from build123d import *

# Parameters (mm, degrees)
CROQUIS1_W              = 304.8
CROQUIS1_H              = 228.6
SALIENTE_EXTRUIR1_DEPTH = 1500
VACIADO1_T              = -2
CROQUIS2_W              = 25.4
CROQUIS2_H              = 228.6
CROQUIS2_W_2            = 304.8
CROQUIS2_H_2            = 25.4
SALIENTE_EXTRUIR2_DEPTH = 2


with BuildPart() as part:
    # Croquis1 → Saliente-Extruir1 (new body)
    with BuildSketch(Plane(origin=(0, 0, 0), x_dir=(1, 0, 0), z_dir=(0, 1, 0))):
        Rectangle(CROQUIS1_W, CROQUIS1_H)
    extrude(amount=SALIENTE_EXTRUIR1_DEPTH)

    # Vaciado1
    vaciado1_openings = [part.faces().sort_by_distance(p)[0] for p in [
        (0, 1500, 0),
        (0, 0, 0),
    ]]
    offset(amount=VACIADO1_T, openings=vaciado1_openings, kind=Kind.INTERSECTION)

    # Croquis2 → Saliente-Extruir2 (add)
    with BuildSketch(Plane(origin=(0, 1500, 0), x_dir=(1, 0, 0), z_dir=(0, 1, 0))):
        with Locations((-165.1, 0)):
            Rectangle(CROQUIS2_W, CROQUIS2_H)
        with Locations((0, 127)):
            Rectangle(CROQUIS2_W_2, CROQUIS2_H_2)
        with Locations((0, -127)):
            Rectangle(CROQUIS2_W_2, CROQUIS2_H_2)
        with Locations((165.1, 0)):
            Rectangle(CROQUIS2_W, CROQUIS2_H)
    saliente_extruir2 = extrude(amount=-SALIENTE_EXTRUIR2_DEPTH)

    # Simetría1: Saliente-Extruir2 across plane
    add(saliente_extruir2.mirror(Plane.ZX.offset(750)))


solid = part.part
CAD build for the part. Positions are in the model's coordinates, mm. A direction names the side the tool comes from. Give positions to 0.01 mm unless a question says otherwise; leave off trailing zeros. Loops run counter-clockwise (first coordinate to the right, second up) from the corner with the lowest first, then second, coordinate; pieces in that order, holes last. Notation, with made-up numbers: M 34.5,-28.5 L 43.5,-28.5 A27 cw 43.5,8.5 Z; hole C -22,5.25 d5. An arc over 180 degrees is marked long. Write each question's results on one line, items separated by ' | '.
Q1. Band-saw the part on C-C on y = 432. Write the cut outline in (x, z).
Geometry check:
outline: M -152.4,-114.3 L 152.4,-114.3 L 152.4,114.3 L -152.4,114.3 Z; hole M -150.4,-112.3 L 150.4,-112.3 L 150.4,112.3 L -150.4,112.3 Z
Q2. Probe probe 1 along Z at (x, y) = (-106.5, 1095.5); probe 2 along X at (y, z) = (127, 27). List the from-to ranges inside material, lowest first.
Geometry check:
probe 1: z = -114.3 to -112.3, 112.3 to 114.3 | probe 2: x = -152.4 to -150.4, 150.4 to 152.4
Q3. Band-saw the part on A-A on z = 64.5. Write the cut outline in (x, y).
Geometry check:
outline: M -177.8,0 L -150.4,0 L -150.4,1500 L -177.8,1500 L -177.8,1498 L -152.4,1498 L -152.4,2 L -177.8,2 Z; M 150.4,0 L 177.8,0 L 177.8,2 L 152.4,2 L 152.4,1498 L 177.8,1498 L 177.8,1500 L 150.4,1500 Z
Q4. Mould opens along X. For faces 1 (the face through (-152.4, 740, 2)), 2 (the face through (-2, 740, 112.3)), 3 (the face through (-2, 2, 127)) say: pulls with the +X half, pulls with the -X half, needs draft (parallel to the pull), parting line crosses it, or undercut.
Geometry check:
face 1: pulls with the -X half | face 2: undercut | face 3: needs draft
Q5. Which spindle directions (+Z, -Z, +X, -X, +Y, -Y) get a long thin tool onto all of the face, cutting with end or side? Do faces 4 (the face through (-2, 740, -114.3)), 5 (the face through (-165, 2, -2)), 6 (the face through (150.4, 740, 2)). Say none if no direction does.
Geometry check:
face 4: -Z, +X, -X | face 5: +Z, -Z, -X | face 6: +Y, -Y
Q6. Flat gauge pins, fed straight in: P1, Ø1, axis at y = 1, z = 130, coming from the +X side; P2, Ø2, axis at x = -88.5, y = 1169.5, coming from the +Z side; P3, Ø7.5, axis at x = -162.5, z = -18.5, coming from the -Y side; P4, Ø6, axis at x = 44.5, y = 1100.5, coming from the -Z side. Where does each tip first touch, or does it go through?
Geometry check:
P1: stops at x = 152.4 | P2: stops at z = 114.3 | P3: stops at y = 0 | P4: stops at z = -114.3
Q7. Band-saw the part on B-B on x = -128.5. Write the cut outline in (y, z), and give its area (3 significant figures).
Geometry check:
outline: M 0,-139.7 L 2,-139.7 L 2,-114.3 L 1498,-114.3 L 1498,-139.7 L 1500,-139.7 L 1500,-112.3 L 0,-112.3 Z; M 0,112.3 L 1500,112.3 L 1500,139.7 L 1498,139.7 L 1498,114.3 L 2,114.3 L 2,139.7 L 0,139.7 Z | area: 6,200 mm²
